Geometry: final body of the model. Coordinates: model frame, mm. A direction names the side the tool comes from. Give positions to 0.01 mm unless a question says otherwise; leave off trailing zeros. Order: outer loops, then holes, each group sorted by start corner. A loop starts at its lowest first (then second) coordinate and runs counter-clockwise, first axis right, second up. Notation, with made-up numbers: (83.25, -25) - (137.25, -25) arc R22 cw to (137.25, 2) - close; hole circle Ø8 at (-26, 36.5). An arc over 180 degrees is marked (long way). Put each result on its own line as item: value. Start each with the question number.
1. Ray query, line 1 along Z through (x, y) = (-21, -2.25); line 2 along Z through (x, y) = (-20, -5.5); line 3 along Z through (x, y) = (-18, -10.75). Return the intervals inside material, ascending. Write a range as from..to.
2. First-contact query: P1, Ø8, axis at x = -3.5, y = -2.5, coming from the +Z side; P2, Ø12, axis at x = -17.5, y = -10.5, coming from the +Z side; P3, Ø12, axis at x = 0.5, y = -10.5, coming from the -Z side. Flat tips, straight axial feed; report the tip coordinate or a pass-through.
3. Section A-A on x = 1.5. Return the cut outline in (y, z), plus the area to 3 significant figures.
4. Set-up query: faces 1 (the flat face through (-15.304, -3, -9)), 2 (the flat face through (-18.304, 0, 0)). Return all of +Z, -Z, +X, -X, +Y, -Y with unobstructed straight access to the full face (end or side cutting, diameter ignored); none if empty.
5. Mould query, pull axis Z, two halves, no side actions, for faces 3 (the flat face through (22.696, 0, 0)), 4 (the flat face through (-21, 0, 2)), 5 (the flat face through (-21, 0, -2)), 6 (the cylindrical face through (2.44, -2.01, -9.03)). Classes: pulls with the +Z half, pulls with the -Z half, needs draft (parallel to the pull), parting line crosses it, or undercut.
from build123d import *

# Parameters (mm, degrees)
F2_W     = 7.449934
F2_H     = 4
F4_DEPTH = 17.733243
F3_R     = 2


with BuildPart() as f1:
    # F0 (on Top) → F1 (revolve)
    with BuildSketch(Plane.XY):
        with BuildLine():
            Line((-25.471063, 0), (22.695719, 0))
            Line((22.695719, 0), (22.695719, 9.25))
            Line((22.695719, 9.25), (-15.304281, 9.25))
            Line((-15.304281, 9.25), (-15.304281, 14.2))
            ThreePointArc((-15.304281, 14.2), (-22.667339, 8.732174), (-25.471063, 0))
        make_face()
    revolve(axis=Axis((-25.471063, 0, 0), (1, 0, 0)))

    # F2 (on Front) → F4 (cut, symmetric)
    with BuildSketch(Plane.XZ):
        with Locations((-22.029248, 0)):
            Rectangle(F2_W, F2_H)
    extrude(amount=F4_DEPTH, both=True, mode=Mode.SUBTRACT)

    # F3
    f3_edges = [f1.edges().sort_by_distance(p)[0] for p in [
        (22.695719, -9.25, 0),
    ]]
    fillet(f3_edges, radius=F3_R)


solid = f1.part
Resolved:
1. line 1: -10.44..-2, 2..10.44
1. line 2: -10.2..-2, 2..10.2
1. line 3: -7.26..7.26
2. P1: z = 9.25
2. P2: z = 13.32
2. P3: z = -8.08
3. outline: circle Ø18.5 at (0, 0)
3. area: 269 mm^2
4. face 1: +X
4. face 2: -X, +Y, -Y
5. face 3: needs draft
5. face 4: undercut
5. face 5: undercut
5. face 6: parting line crosses it
